Design review of the part built by this model. Coordinates are the model's own, in mm. A direction names the side the tool comes from. Give positions to 0.01 mm unless a question says otherwise; leave off trailing zeros. Write each loop counter-clockwise with the first axis right and the second up, starting at its lowest first coordinate (ties: lowest second). Pieces come first, ordered by that corner, then holes. Notation, with made-up numbers: M 62.5,-28 L 67.5,-28 A20 cw 67.5,-14 Z; hole C 49.25,73.5 d5. An arc over 180 degrees is marked long. Answer in a Markdown table with one row per item.
```python
from build123d import *

# Parameters (mm, degrees)
SKETCH1_W      = 23
SKETCH1_H      = 9
EXTRUDE1_DEPTH = 19
SKETCH2_R      = 1.6
EXTRUDE2_DEPTH = 23.888930821
SKETCH3_W      = 19.5
SKETCH3_H      = 15
EXTRUDE3_DEPTH = 25.02759827
SKETCH6_R      = 1.6
EXTRUDE4_DEPTH = 3
EXTRUDE5_START = 3
SKETCH7_R      = 1.6
EXTRUDE5_DEPTH = 3
FILLET1_R      = 2
SKETCH8_W      = 1.59
SKETCH8_H      = 4
EXTRUDE6_DEPTH = 6
SKETCH9_W      = 1.19
SKETCH9_H      = 3.6
EXTRUDE7_DEPTH = 24.072179755


with BuildPart() as part:
    # Sketch1 → Extrude1 (new body)
    with BuildSketch(Plane(origin=(0, 0, 0), x_dir=(1, 0, 0), z_dir=(0, 1, 0))):
        with Locations((-0.132947977, 0.751445087)):
            Rectangle(SKETCH1_W, SKETCH1_H)
    extrude(amount=EXTRUDE1_DEPTH)

    # Sketch2 → Extrude2 (cut, through all)
    with BuildSketch(Plane(origin=(0, 19, 0), x_dir=(1, 0, 0), z_dir=(0, 1, 0))):
        with Locations(Location((-0.632947977, 0.751445087, 0), (0, 0, 270))):
            Circle(SKETCH2_R)
    extrude(amount=-EXTRUDE2_DEPTH, mode=Mode.SUBTRACT)

    # Sketch3 → Extrude3 (cut, through all)
    with BuildSketch(Plane.XY.offset(3.748554913)):
        with Locations((-1.882947977, 9.5)):
            Rectangle(SKETCH3_W, SKETCH3_H)
    extrude(amount=-EXTRUDE3_DEPTH, mode=Mode.SUBTRACT)

    # Sketch6 → Extrude4 (add)
    with BuildSketch(Plane(origin=(0, 2, 0), x_dir=(1, 0, 0), z_dir=(0, 1, 0))):
        with Locations(Location((-6.132947977, 0.751445087, 0), (0, 0, 90))):
            Circle(SKETCH6_R)
    extrude(amount=EXTRUDE4_DEPTH)

    # Sketch7 → Extrude5 (add)
    with BuildSketch(Plane.XZ.offset(-17).offset(EXTRUDE5_START)):
        with Locations(Location((-6.132947977, -0.751445087, 0), (0, 0, 270))):
            Circle(SKETCH7_R)
    extrude(amount=-EXTRUDE5_DEPTH)

    # Fillet1
    fillet1_edges = [part.edges().sort_by_distance(p)[0] for p in [
        (11.367052023, 19, -0.751445087),
        (-0.132947977, 19, -5.251445087),
        (7.867052023, 2, -0.751445087),
        (7.867052023, 17, -0.751445087),
        (-11.632947977, 19, -0.751445087),
        (-0.132947977, 0, -5.251445087),
        (11.367052023, 0, -0.751445087),
        (-0.132947977, 0, 3.748554913),
        (-11.632947977, 0, -0.751445087),
        (-0.132947977, 19, 3.748554913),
        (11.367052023, 9.5, -5.251445087),
        (11.367052023, 9.5, 3.748554913),
    ]]
    fillet(fillet1_edges, radius=FILLET1_R - 0.0001)  # a hair under: the kernel refuses the full size

    # Sketch8 → Extrude6 (cut)
    with BuildSketch(Plane.XY.offset(3.748554913)):
        with Locations((9.572052023, 9.5)):
            Rectangle(SKETCH8_W, SKETCH8_H)
    extrude(amount=-EXTRUDE6_DEPTH, mode=Mode.SUBTRACT)

    # Sketch9 → Extrude7 (cut, through all)
    with BuildSketch(Plane.XY.offset(-2.251445087)):
        with Locations((9.572052023, 9.5)):
            Rectangle(SKETCH9_W, SKETCH9_H)
    extrude(amount=-EXTRUDE7_DEPTH, mode=Mode.SUBTRACT)


solid = part.part
```
1) The part is to be moulded in two halves that separate along X. For faces 6 (the face through (10.797, 18.399, -0.786)), 7 (the face through (-4.57, 3.48, -0.4)), 8 (the face through (-0.99, 0.57, -4.65)), say which applies: released by +X, released by -X, zero draft, split by the parting line, or undercut.
Geometry says:
| item | result |
|---|---|
| face 6 | released by +X |
| face 7 | undercut |
| face 8 | zero draft |
2) Add section B-B (z = -1.25). Count the separate pieces of the cut face and the enclosed holes in it, and give its area (3 significant figures).
Geometry says:
| item | result |
|---|---|
| separate pieces | 3 |
| enclosed holes | 1 |
| area | 143 mm^2 |
3) Insertion check: P1, Ø1.7, axis at x = 9.5, y = 10, coming from the +Z side; P2, Ø2, axis at y = 11, z = -2, coming from the -X side; P3, Ø1, axis at y = 3, z = 2.5, coming from the -X side; P4, Ø8, axis at x = -2, y = 12.5, coming from the +Z side. Each pin has a flat end and moves straight along its axis. Give the tip position at first contact, or say it passes through.
Geometry says:
| item | result |
|---|---|
| P1 | z = 3.75 |
| P2 | x = 7.87 |
| P3 | x = 7.19 |
| P4 | z = 0.79 |
4) For faces 1 (the face through (10.167, 9, -4)), 2 (the face through (-4.547, 15.479, -0.543)), 3 (the face through (10, 11.5, 1)), 4 (the face through (10.766, 9.605, -4.681)), 5 (the face through (-11.03, 18.43, -0.81)), list the 3-axis set-ups (+Z, -Z, +X, -X, +Y, -Y) from which the entire face can be reached by the end or side of a thin tool; tool diameter is ignored.
Geometry says:
| item | result |
|---|---|
| face 1 | +Z, -Z |
| face 2 | none |
| face 3 | +Z |
| face 4 | -Z, +X, +Y, -Y |
| face 5 | +Z, -Z, -X, +Y |
5) To check wall thickness, follow probe 1 along Y at (x, z) = (9, -1.75); probe 2 along Y at (x, z) = (-9.75, 0.5); probe 3 along X at (y, z) = (9.75, 1.75). State the ranges of each line that lie inside material, in increasing order. Write a range as [from, to].
Geometry says:
| item | result |
|---|---|
| probe 1 | [0, 7.5], [11.5, 19] |
| probe 2 | [0, 2], [17, 19] |
| probe 3 | [7.87, 8.78], [10.37, 11.37] |
6) Add section A-A (y = 11). Write out the cut boundary in (x, z).
Geometry says:
| item | result |
|---|---|
| outline | M 7.87,-5.25 L 8.98,-5.25 L 8.98,-2.25 L 8.78,-2.25 L 8.78,3.75 L 7.87,3.75 Z; M 10.17,-5.08 A2 ccw 11.37,-3.25 L 11.37,1.75 A2 ccw 10.37,3.48 L 10.37,-2.25 L 10.17,-2.25 Z |
